from build123d import *

# Parameters (mm, degrees)
BOSS_EXTRUDE1_DEPTH      = 5
CUT_EXTRUDE1_DEPTH       = 1.5
CUT_EXTRUDE2_DEPTH       = 1.5
F_4_0_4_DIAMETER_HOLE1_D = 4
BOSS_EXTRUDE2_START      = -5
SKETCH6_R                = 4
BOSS_EXTRUDE2_DEPTH      = 5
SKETCH7_R                = 2
CUT_EXTRUDE3_DEPTH       = 56.788378253


with BuildPart() as part:
    # Sketch1 → Boss-Extrude1 (new body)
    with BuildSketch(Plane(origin=(0, 0, 0), x_dir=(-1, 0, 0), z_dir=(0, 0, -1))):
        with BuildLine():
            Line((0, 4), (-51.4197, 4))
            ThreePointArc((-51.4197, 4), (-55.4197, 0), (-51.4197, -4))
            Line((-51.4197, -4), (0, -4))
            ThreePointArc((0, -4), (4, 0), (0, 4))
        make_face()
    extrude(amount=-BOSS_EXTRUDE1_DEPTH)

    # Sketch2 → Cut-Extrude1 (cut)
    with BuildSketch(Plane(origin=(0, 0, 0), x_dir=(-1, 0, 0), z_dir=(0, 0, -1))):
        with BuildLine():
            Line((-6, 2.5), (-45.4197, 2.5))
            ThreePointArc((-45.4197, 2.5), (-47.9197, 0), (-45.4197, -2.5))
            Line((-45.4197, -2.5), (-6, -2.5))
            ThreePointArc((-6, -2.5), (-3.5, 0), (-6, 2.5))
        make_face()
    extrude(amount=-CUT_EXTRUDE1_DEPTH, mode=Mode.SUBTRACT)

    # Sketch3 → Cut-Extrude2 (cut)
    with BuildSketch(Plane.XY.offset(5)):
        with BuildLine():
            Line((6, -2), (45.4197, -2))
            ThreePointArc((45.4197, -2), (47.4197, 0), (45.4197, 2))
            Line((45.4197, 2), (6, 2))
            ThreePointArc((6, 2), (4, 0), (6, -2))
        make_face()
    extrude(amount=-CUT_EXTRUDE2_DEPTH, mode=Mode.SUBTRACT)

    # Ø4.0 (4) Diameter Hole1 (through all)
    with Locations(Plane(origin=(0, 0, 0), x_dir=(-1, 0, 0), z_dir=(0, 0, -1))):
        with Locations((-51.4197, 0), (0, 0)):
            Hole(F_4_0_4_DIAMETER_HOLE1_D / 2)

    # Sketch6 → Boss-Extrude2 (add)
    with BuildSketch(Plane.XY.offset(5).offset(BOSS_EXTRUDE2_START)):
        with Locations((25.70985, 0)):
            Circle(SKETCH6_R)
    extrude(amount=BOSS_EXTRUDE2_DEPTH)

    # Sketch7 → Cut-Extrude3 (cut, through all)
    with BuildSketch(Plane.XY.offset(5)):
        with Locations((25.70985, 0)):
            Circle(SKETCH7_R)
    extrude(amount=-CUT_EXTRUDE3_DEPTH, mode=Mode.SUBTRACT)


solid = part.part
Build history of the part. All positions in model axes, mm. A direction names the side the tool comes from. Round coordinates to 2 decimals unless told otherwise and drop trailing zeros. Write each loop counter-clockwise with the first axis right and the second up, starting at its lowest first coordinate (ties: lowest second). Pieces come first, ordered by that corner, then holes. Notation, with made-up numbers: M -17.75,25 L -8.75,25 A15 cw -8.75,43 Z; hole C 23,55 d6. An arc over 180 degrees is marked long. Answer in a Markdown table with one row per item.
1. Saw through at A-A (y = 0). State how many separate pieces and enclosed holes the cut face has, and give its area (3 significant figures).
Geometry check:
| item | result |
|---|---|
| separate pieces | 4 |
| enclosed holes | 0 |
| area | 129 mm2 |
2. Probe L1, parallel to Y at x = 17.5, z = 0.7; L2, parallel to X at y = -0.5, z = 0.2; L3, parallel to Y at x = 0, z = 2.45. List the from-to ranges inside material, lowest first. Write a range as [from, to].
Geometry check:
| item | result |
|---|---|
| L1 | [-4, -2.5], [2.5, 4] |
| L2 | [-3.97, -1.94], [1.94, 3.55], [21.74, 23.77], [27.65, 29.68], [47.87, 49.48], [53.36, 55.39] |
| L3 | [-4, -2], [2, 4] |
3. Which spindle directions (+Z, -Z, +X, -X, +Y, -Y) get a long thin tool onto all of the face, cutting with end or side? Do faces 5 (the face through (13, 0, 3.5)), 6 (the face through (0, -2, 3)), 7 (the face through (3.5, -0.1, 0.7)). Say none if no direction does.
Geometry check:
| item | result |
|---|---|
| face 5 | +Z |
| face 6 | +Z, -Z |
| face 7 | -Z |
4. Mould opens along X. For faces 1 (the face through (14, 2, 4)), 2 (the face through (25, 4, 2)), 3 (the face through (49.42, 0.09, 2.53)), 4 (the face through (55.42, 0.09, 2.46)) say: +X half, -X half, draft (parallel to the pull), parting line (faces both ways), or undercut.
Geometry check:
| item | result |
|---|---|
| face 1 | undercut |
| face 2 | draft |
| face 3 | undercut |
| face 4 | +X half |
5. Saw through at C-C (x = 37). List the corners of the cut face in (y, z).
Geometry check:
| item | result |
|---|---|
| outline | M -4,0 L -2.5,0 L -2.5,1.5 L 2.5,1.5 L 2.5,0 L 4,0 L 4,5 L 2,5 L 2,3.5 L -2,3.5 L -2,5 L -4,5 Z |
6. Saw through at D-D (y = 3). List the corners of the cut face in (x, z).
Geometry check:
| item | result |
|---|---|
| outline | M -2.65,0 L 54.07,0 L 54.07,5 L -2.65,5 Z |
7. Flat gauge pins, fed straight in: P1, Ø1.5, axis at x = 34, y = 1.5, coming from the -Z side; P2, Ø1.5, axis at y = -3, z = 4, coming from the -X side. Where does each tip first touch, or does it go through?
Geometry check:
| item | result |
|---|---|
| P1 | z = 1.5 |
| P2 | x = -3.31 |
8. Saw through at B-B (z = 2.85). List the corners of the cut face in (x, y).
Geometry check:
| item | result |
|---|---|
| outline | M 0,-4 L 51.42,-4 A4 ccw 51.42,4 L 0,4 A4 ccw Z; hole C 0,0 d4; hole C 25.71,0 d4; hole C 51.42,0 d4 |
